Can you work these out from the model? Positions are in its coordinate system, mm. A direction names the side the tool comes from. Coordinates: 2 decimals unless noted, no trailing zeros. Order: outer loops, then holes, each group sorted by start corner. A loop starts at its lowest first (then second) coordinate and runs counter-clockwise, first axis right, second up. Notation, with made-up numbers: (-29, 85.5) -> (30, 85.5) arc R31 cw to (30, 110.5) -> close; hole circle Ø3 at (-37.5, 62.25). An arc over 180 degrees is marked (long way). Answer as a JSON object with one key per item and string values. Group by question number.
(1) I want a section at B-B, the plane y = 16.5. List the corners of the cut face in (x, z) for me.
(2) I want a section at D-D, the plane z = -11.5. List the corners of the cut face in (x, y) for me, plus the area to 3 significant figures.
(3) I want a section at C-C, the plane x = -5. List the corners of the cut face in (y, z) for me.
(4) If we mould it in two halves opening along Z, with no side actions, what happens to faces 5 (the flat face through (0, -16, 61.5)), 6 (the flat face through (-31, -10, 16.5)), 7 (the flat face through (16.5, 1, 47))? For each: pulls with the +Z half, pulls with the -Z half, needs draft (parallel to the pull), parting line crosses it, or undercut.
(5) I need wall thicknesses on line 1 (X direction, y = -25, z = -12); line 2 (Z direction, x = -8.5, y = -7); line 3 (Y direction, x = 26, z = -4.5). Which ranges of each line are inside material? Lowest first, please.
(6) For pin 1 (3 mm diameter, centred on x = -16, y = 5.5, fed in from +Z); pin 2 (1.5 mm diameter, centred on y = 28.5, z = 13.5, fed in from -X); pin 3 (6 mm diameter, centred on y = 5, z = -41, fed in from +X); pin 4 (13 mm diameter, centred on x = 10.5, y = 11.5, fed in from +Z), each with a flat end and sliding along its axis, tell me the tip position at first contact or that it passes through.
(7) I want a section at A-A, the plane y = -26. List the corners of the cut face in (x, z) for me, plus the area to 3 significant figures.
(8) Which directions (+Z, -Z, +X, -X, +Y, -Y) give clear straight access to the entire face, cutting with the end or side of a thin tool? Please do faces 1 (the flat face through (16.5, 1, -47)), 2 (the flat face through (-31, -10, -16.5)), 3 (the flat face through (31, -8, 16.5)), 4 (the flat face through (12, 17, 25)).
from build123d import *

# Parameters (mm, degrees)
F0_W     = 33
F0_H     = 47
F0_W_2   = 15.5
F0_H_2   = 33
F1_DEPTH = 3
F2_W     = 33
F2_H     = 2
F2_W_2   = 2
F2_H_2   = 33
F3_DEPTH = 33
F5_DEPTH = 25


with BuildPart() as f1:
    # F0 (on Front) → F1 (new body)
    with BuildSketch(Plane.XZ):
        with Locations((0, 40)):
            Rectangle(F0_W, F0_H)
        with Locations((24.25, 0)):
            Rectangle(F0_W_2, F0_H_2)
        Rectangle(F0_W, F0_H_2)
        with Locations((-24.25, 0)):
            Rectangle(F0_W_2, F0_H_2)
        with Locations((0, -40)):
            Rectangle(F0_W, F0_H)
    extrude(amount=-F1_DEPTH)

    # F2 (on face) → F3 (join)
    with BuildSketch(Plane.XZ):
        with Locations((0, 62.5)):
            Rectangle(F2_W, F2_H)
        with Locations((-31, 0)):
            Rectangle(F2_W_2, F2_H_2)
        with Locations((0, -62.5)):
            Rectangle(F2_W, F2_H)
        with Locations((31, 0)):
            Rectangle(F2_W_2, F2_H_2)
    extrude(amount=F3_DEPTH)

    # F4 (on Top) → F5 (join)
    with BuildSketch(Plane.XY):
        with BuildLine():
            Line((-11.8321595662, 3), (0, 3))
            ThreePointArc((0, 3), (-11.4000157684, 12.9868441982), (-3, 25.6018016556))
            Line((-3, 25.6018016556), (-3, 30.7249807396))
            ThreePointArc((-3, 30.7249807396), (-15.7215418646, 19.5083052421), (-11.8321595662, 3))
        make_face()
        with BuildLine():
            ThreePointArc((3, 25.6018016556), (9.1309911839, 21.4910657271), (11.5, 14.5))
            ThreePointArc((11.5, 14.5), (8.1317279836, 6.3682720164), (0, 3))
            Line((0, 3), (11.8321595662, 3))
            ThreePointArc((11.8321595662, 3), (15.2885681612, 8.294382901), (16.5, 14.5))
            ThreePointArc((16.5, 14.5), (12.683650894, 25.0534354596), (3, 30.7249807396))
            Line((3, 30.7249807396), (3, 25.6018016556))
        make_face()
    extrude(amount=F5_DEPTH)


solid = f1.part
Computed values:
{
 "1": {"outline": "(-16.38, 0) -> (-11.32, 0) -> (-11.32, 25) -> (-16.38, 25) -> close; (11.32, 0) -> (16.38, 0) -> (16.38, 25) -> (11.32, 25) -> close"},
 "2": {"outline": "(-32, -33) -> (-30, -33) -> (-30, 0) -> (30, 0) -> (30, -33) -> (32, -33) -> (32, 3) -> (-32, 3) -> close", "area": "324 mm2"},
 "3": {"outline": "(-33, -63.5) -> (3, -63.5) -> (3, 0) -> (4.14, 0) -> (4.14, 25) -> (3, 25) -> (3, 63.5) -> (-33, 63.5) -> (-33, 61.5) -> (0, 61.5) -> (0, -61.5) -> (-33, -61.5) -> close; (24.86, 0) -> (30.22, 0) -> (30.22, 25) -> (24.86, 25) -> close"},
 "4": {"face 5": "undercut", "face 6": "pulls with the +Z half", "face 7": "needs draft"},
 "5": {"line 1": "x = -32 to -30, 30 to 32", "line 2": "z = -63.5 to -61.5, 61.5 to 63.5", "line 3": "y = 0 to 3"},
 "6": {"pin 1": "passes through", "pin 2": "stops at x = -9.83", "pin 3": "stops at x = 16.5", "pin 4": "stops at z = 25"},
 "7": {"outline": "(-32, -16.5) -> (-30, -16.5) -> (-30, 16.5) -> (-32, 16.5) -> close; (-16.5, -63.5) -> (16.5, -63.5) -> (16.5, -61.5) -> (-16.5, -61.5) -> close; (-16.5, 61.5) -> (16.5, 61.5) -> (16.5, 63.5) -> (-16.5, 63.5) -> close; (30, -16.5) -> (32, -16.5) -> (32, 16.5) -> (30, 16.5) -> close", "area": "264 mm2"},
 "8": {"face 1": "-Z, +X, +Y, -Y", "face 2": "-Z, -X, +Y, -Y", "face 3": "+Z, +X, +Y, -Y", "face 4": "+Z, +X, -X, +Y"}
}
